Input: part model. Units: mm. Frame: model coordinates. Give positions to 0.01 mm unless a question says otherwise; leave off trailing zeros. Loops run counter-clockwise (first coordinate to the right, second up) from the corner with the lowest first, then second, coordinate; pieces in that order, holes last. Notation, with made-up numbers: M 80.5,-17.5 L 137.5,-17.5 A34 ccw 137.5,20.5 Z; hole C -1.75,45.25 d10. An arc over 180 degrees is marked long. Answer as a JSON object with one key per item and string values. Group by question number.
```python
from build123d import *

# Parameters (mm, degrees)
SKETCH1_W           = 15
SKETCH1_H           = 18
SKETCH1_R           = 1.5
BOSS_EXTRUDE1_DEPTH = 4
FILLET1_R           = 3
CUT_EXTRUDE2_DEPTH  = 24.769728648
LPATTERN1_COUNT     = 10
LPATTERN1_PITCH     = 2


with BuildPart() as part:
    # Sketch1 → Boss-Extrude1 (new body)
    with BuildSketch(Plane.XY):
        with Locations((7.5, 9)):
            Rectangle(SKETCH1_W, SKETCH1_H)
        with Locations((7.5, 9)):
            Circle(SKETCH1_R, mode=Mode.SUBTRACT)
    extrude(amount=BOSS_EXTRUDE1_DEPTH)

    # Fillet1
    fillet1_edges = [part.edges().sort_by_distance(p)[0] for p in [
        (15, 9, 0),
    ]]
    fillet(fillet1_edges, radius=FILLET1_R)

    # Sketch2 → Cut-Extrude2 (cut, through all)
    with BuildSketch(Plane(origin=(0, 0, 0), x_dir=(1, 0, 0), z_dir=(0, 1, 0))):
        with BuildLine():
            Line((-1, 0), (1, 0))
            ThreePointArc((1, 0), (0.6875, -0.104166667), (0.5, -0.375))
            ThreePointArc((0.5, -0.375), (0, -0.75), (-0.5, -0.375))
            ThreePointArc((-0.5, -0.375), (-0.6875, -0.104166667), (-1, 0))
        make_face()
    cut_extrude2 = extrude(amount=CUT_EXTRUDE2_DEPTH, mode=Mode.SUBTRACT)

    # LPattern1: Cut-Extrude2 ×10
    with Locations(*[(i * LPATTERN1_PITCH, 0, 0) for i in range(1, LPATTERN1_COUNT)]):
        add(cut_extrude2, mode=Mode.SUBTRACT)


solid = part.part
```
1. Mould query, pull axis X, two halves, no side actions, for faces 1 (the cylindrical face through (9, 9, 2)), 2 (the flat face through (7, 18, 2)), 3 (the flat face through (0, 9, 2)), 4 (the flat face through (15, 8.9, 3.5)). Classes: pulls with the +X half, pulls with the -X half, needs draft (parallel to the pull), parting line crosses it, or undercut.
2. Material intervals for L1, parallel to Y at x = 7.5, z = 1.8; L2, parallel to Y at x = 8.5, z = 2.75; L3, parallel to X at y = 8.75, z = 1.55, sorted ascending.
3. Section B-B (z = 3.35). Output: boundary loops of the cut face in (x, y), then the cut area to 3 significant figures.
4. Section A-A (y = 11.75). Output: boundary loops of the cut face in (x, z) (3 decimals), then the cut area to 3 significant figures.
5. Section C-C (x = 11.25). Output: boundary loops of the cut face in (y, z), then the cut area to 3 significant figures.
Geometry results:
{
 "1": {"face 1": "undercut", "face 2": "needs draft", "face 3": "pulls with the -X half", "face 4": "pulls with the +X half"},
 "2": {"L1": "0 to 7.5, 10.5 to 18", "L2": "0 to 7.88, 10.12 to 18", "L3": "0 to 6.02, 8.98 to 14.63"},
 "3": {"outline": "M 0,0 L 15,0 L 15,18 L 0,18 Z; hole C 7.5,9 d3", "area": "263 mm2"},
 "4": {"outline": "M 0,0.75 A0.521 cw 0.5,0.375 A0.521 ccw 1.5,0.375 A0.521 cw 2.5,0.375 A0.521 ccw 3.5,0.375 A0.521 cw 4.5,0.375 A0.521 ccw 5.5,0.375 A0.521 cw 6.5,0.375 A0.521 ccw 7.5,0.375 A0.521 cw 8.5,0.375 A0.521 ccw 9.5,0.375 A0.521 cw 10.5,0.375 A0.521 ccw 11.5,0.375 A0.521 cw 12.5,0.375 A0.521 ccw 12.713,0.086 A3 ccw 13.511,0.408 A0.521 cw 13.984,0.75 A3 ccw 15,3 L 15,4 L 0,4 Z", "area": "53.2 mm2"},
 "5": {"outline": "M 0,0.06 L 18,0.06 L 18,4 L 0,4 Z", "area": "70.8 mm2"}
}
